Study the drawing (mm; zero at the part's minimum x, y, z) and answer. Round coordinates to 2 decimals unless told otherwise and drop trailing zeros. Loops run counter-clockwise (first coordinate to the right, second up) from the corner with the lowest first, then second, coordinate; pieces in that order, holes last. Notation, with made-up numbers: (-23, 14) -> (-11, 14) arc R26 ccw to (-11, 36) -> close; hole circle Ø11 at (10.5, 63). An arc over 180 degrees is marked (long way). Write each question's results on one line, items separated by ' | '. Start each with the question number.
(1) The part is cut by section A-A (x = 31). Determine the outline of the cut face in (y, z), plus the area to 3 significant figures.
(2) Determine the mould class of the marked faces 1, 2, 3 and 4 for opening direction X: released by +X, released by -X, zero draft, split by the parting line, or undercut.
(3) The part is cut by section D-D (y = 58). Determine the outline of the cut face in (x, z).
(4) Flat-ended cylindrical pins translate along their axes: pin 1 (4 mm diameter, centred on x = 16, y = 29, fed in from +Z); pin 2 (1 mm diameter, centred on y = 41.5, z = 5.5, fed in from -X); pin 3 (1.5 mm diameter, centred on x = 52, z = 8, fed in from -Y). Find the tip coordinate at first contact, or state that the pin passes through.
(5) Straight lines are drawn through the part: probe 1 along Y at (x, z) = (31, 4.5); probe 2 along Y at (x, z) = (31, 11.35); probe 3 along Z at (x, y) = (3, 21). For each, find the intervals that lie inside material, in ascending order.
(6) The part is cut by section C-C (z = 4). Determine the outline of the cut face in (x, y).
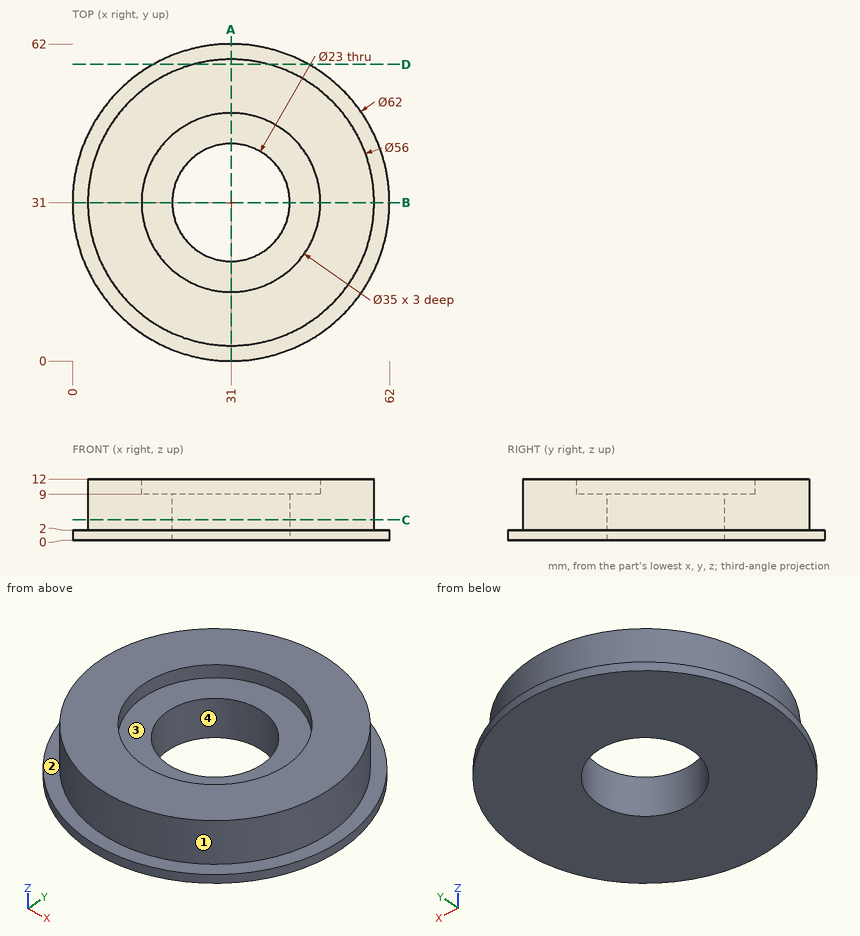
Checked values:
1) outline: (0, 0) -> (19.5, 0) -> (19.5, 9) -> (13.5, 9) -> (13.5, 12) -> (3, 12) -> (3, 2) -> (0, 2) -> close; (42.5, 0) -> (62, 0) -> (62, 2) -> (59, 2) -> (59, 12) -> (48.5, 12) -> (48.5, 9) -> (42.5, 9) -> close | area: 372 mm2
2) face 1: split by the parting line | face 2: zero draft | face 3: undercut | face 4: undercut
3) outline: (15.77, 0) -> (46.23, 0) -> (46.23, 2) -> (38.42, 2) -> (38.42, 12) -> (23.58, 12) -> (23.58, 2) -> (15.77, 2) -> close
4) pin 1: stops at z = 9 | pin 2: stops at x = 4.85 | pin 3: stops at y = 11.66
5) probe 1: y = 3 to 19.5, 42.5 to 59 | probe 2: y = 3 to 13.5, 48.5 to 59 | probe 3: z = 0 to 2
6) outline: circle Ø56 at (31, 31); hole circle Ø23 at (31, 31)
